```python
from build123d import *

# Parameters (mm, degrees)
SKIZZE1_R                       = 1.75
AUFSATZ_LINEAR_AUSTRAGEN1_DEPTH = 29
SKIZZE2_W                       = 95.177468056
SKIZZE2_H                       = 43
SCHNITT_LINEAR_AUSTRAGEN1_DEPTH = 29
SKIZZE5_W                       = 102.378587485
SKIZZE5_H                       = 44.26226899
SCHNITT_LINEAR_AUSTRAGEN2_DEPTH = 29
SKIZZE6_W                       = 21
SKIZZE6_H                       = 11
SCHNITT_LINEAR_AUSTRAGEN3_DEPTH = 2
SKIZZE7_R                       = 3
SCHNITT_LINEAR_AUSTRAGEN4_DEPTH = 2
SKIZZE8_R                       = 1.75
SCHNITT_LINEAR_AUSTRAGEN5_DEPTH = 102.965680501


with BuildPart() as part:
    # Skizze1 → Aufsatz-Linear austragen1 (new body)
    with BuildSketch(Plane.XY):
        with BuildLine():
            Line((31, -13.5), (31, 0.5))
            ThreePointArc((31, 0.5), (30.121320344, 2.621320344), (28, 3.5))
            Line((28, 3.5), (-15, 3.5))
            ThreePointArc((-15, 3.5), (-21.363961031, 6.136038969), (-24, 12.5))
            Line((-24, 12.5), (-24, 30.5))
            ThreePointArc((-24, 30.5), (-24.878679656, 32.621320344), (-27, 33.5))
            Line((-27, 33.5), (-81, 33.5))
            ThreePointArc((-81, 33.5), (-83.121320344, 32.621320344), (-84, 30.5))
            Line((-84, 30.5), (-84, 29.5))
            ThreePointArc((-84, 29.5), (-83.121320344, 27.378679656), (-81, 26.5))
            Line((-81, 26.5), (-36, 26.5))
            ThreePointArc((-36, 26.5), (-32.464466094, 25.035533906), (-31, 21.5))
            Line((-31, 21.5), (-31, 5.5))
            ThreePointArc((-31, 5.5), (-28.363961031, -0.863961031), (-22, -3.5))
            Line((-22, -3.5), (18, -3.5))
            ThreePointArc((18, -3.5), (20.121320344, -4.378679656), (21, -6.5))
            Line((21, -6.5), (21, -13.5))
            ThreePointArc((21, -13.5), (21.878679656, -15.621320344), (24, -16.5))
            Line((24, -16.5), (28, -16.5))
            ThreePointArc((28, -16.5), (30.121320344, -15.621320344), (31, -13.5))
        make_face()
        with Locations(Location((26, -1.150447614, 0), (0, 0, 180))):
            Circle(SKIZZE1_R, mode=Mode.SUBTRACT)
        with Locations(Location((26, -11.849552386, 0), (0, 0, 180))):
            Circle(SKIZZE1_R, mode=Mode.SUBTRACT)
    extrude(amount=AUFSATZ_LINEAR_AUSTRAGEN1_DEPTH)

    # Skizze2 → Schnitt-Linear austragen1 (cut)
    with BuildSketch(Plane.XY.offset(24.5)):
        with Locations((-3.395581908, 5)):
            Rectangle(SKIZZE2_W, SKIZZE2_H)
    extrude(amount=SCHNITT_LINEAR_AUSTRAGEN1_DEPTH, mode=Mode.SUBTRACT)

    # Skizze5 → Schnitt-Linear austragen2 (cut)
    with BuildSketch(Plane.XY.offset(17.5)):
        with Locations((-5.60029533, 4.368865505)):
            Rectangle(SKIZZE5_W, SKIZZE5_H)
    extrude(amount=-SCHNITT_LINEAR_AUSTRAGEN2_DEPTH, mode=Mode.SUBTRACT)

    # Skizze6 → Schnitt-Linear austragen3 (cut)
    with BuildSketch(Plane(origin=(0, 33.5, 0), x_dir=(1, 0, 0), z_dir=(0, 1, 0))):
        with Locations((-54, -7.342518692)):
            Rectangle(SKIZZE6_W, SKIZZE6_H)
        with Locations((-54, -21.657481308)):
            Rectangle(SKIZZE6_W, SKIZZE6_H)
    extrude(amount=-SCHNITT_LINEAR_AUSTRAGEN3_DEPTH, mode=Mode.SUBTRACT)

    # Skizze7 → Schnitt-Linear austragen4 (cut)
    with BuildSketch(Plane.XY.offset(24.5)):
        with Locations((26, -1.150447614)):
            Circle(SKIZZE7_R)
        with Locations((26, -11.849552386)):
            Circle(SKIZZE7_R)
    extrude(amount=-SCHNITT_LINEAR_AUSTRAGEN4_DEPTH, mode=Mode.SUBTRACT)

    # Skizze8 → Schnitt-Linear austragen5 (cut, through all)
    with BuildSketch(Plane(origin=(0, 33.5, 0), x_dir=(1, 0, 0), z_dir=(0, 1, 0))):
        with Locations(Location((-54, -7.342518692, 0), (0, 0, 270))):
            Circle(SKIZZE8_R)
        with Locations(Location((-54, -21.657481308, 0), (0, 0, 90))):
            Circle(SKIZZE8_R)
    extrude(amount=-SCHNITT_LINEAR_AUSTRAGEN5_DEPTH, mode=Mode.SUBTRACT)


solid = part.part
```
For this review, take the finished solid that the model builds, in its own axes (mm). A direction names the side the tool comes from. Give positions to 0.01 mm unless a question says otherwise; leave off trailing zeros. Order: outer loops, then holes, each group sorted by start corner. A loop starts at its lowest first (then second) coordinate and runs counter-clockwise, first axis right, second up.
1) Take a section at D-D (y = 28). Give the boundary of the cut face in (x, z).
2) For faces 1 (the face through (-54, 33.5, 14)), 2 (the face through (26, -3.1, 22.5)), 3 (the face through (-31, 14, 21)), 4 (the face through (-64.5, 33, 22)), list the 3-axis set-ups (+Z, -Z, +X, -X, +Y, -Y) from which the entire face can be reached by the end or side of a thin tool; tool diameter is ignored.
3) Take a section at B-B (z = 7.25). Give the boundary of the cut face in (x, y).
4) The part is to be moulded in two halves that separate along X. For faces 5 (the face through (-43.5, 33, 7)), 6 (the face through (7, 3.5, 21)), 7 (the face through (-83.1, 32.64, 14.3)), say which applies: released by +X, released by -X, zero draft, split by the parting line, or undercut.
5) Take a section at A-A (x = 26). Give the boundary of the cut face in (y, z).
6) Wall thickness on line 1 (Y direction, x = 26, z = 19.45); line 2 (Y direction, x = 26, z = 23.9); line 3 (Z direction, x = -28, y = 5.5): over which ranges is each line inside the solid? List them lowest first.
7) Take a section at C-C (x = -54). Give the boundary of the cut face in (y, z), then the cut area to 3 significant figures.
8) Insertion check: pin 1 (1.5 mm diameter, centred on x = -67, z = 17.5, fed in from -Y); pin 2 (6 mm diameter, centred on x = -30, y = 8, fed in from -Z); pin 3 (5 mm diameter, centred on y = 24.5, z = 21, fed in from -X). Each pin has a flat end and moves straight along its axis. Give the tip position at first contact, or say it passes through.
Derived:
1. outline: (-83.6, 0) - (-24, 0) - (-24, 29) - (-83.6, 29) - close; hole circle Ø3.5 at (-54, 7.34); hole circle Ø3.5 at (-54, 21.66)
2. face 1: +Z, -Z, +X, -X, +Y
2. face 2: +Z
2. face 3: +Z, -Z, -X, -Y
2. face 4: +Y
3. outline: (-84, 29.5) arc R3 ccw to (-81, 26.5) - (-55.75, 26.5) - (-55.75, 31.5) - (-64.5, 31.5) - (-64.5, 33.5) - (-81, 33.5) arc R3 ccw to (-84, 30.5) - close; (-52.25, 26.5) - (-24, 26.5) - (-24, 30.5) arc R3 ccw to (-27, 33.5) - (-43.5, 33.5) - (-43.5, 31.5) - (-52.25, 31.5) - close
4. face 5: undercut
4. face 6: zero draft
4. face 7: released by -X
5. outline: (-16.5, 17.5) - (-13.6, 17.5) - (-13.6, 22.5) - (-14.85, 22.5) - (-14.85, 24.5) - (-16.5, 24.5) - close; (-10.1, 17.5) - (-2.9, 17.5) - (-2.9, 22.5) - (-4.15, 22.5) - (-4.15, 24.5) - (-8.85, 24.5) - (-8.85, 22.5) - (-10.1, 22.5) - close; (0.6, 17.5) - (3.5, 17.5) - (3.5, 24.5) - (1.85, 24.5) - (1.85, 22.5) - (0.6, 22.5) - close
6. line 1: y = -16.5 to -13.6, -10.1 to -2.9, 0.6 to 3.5
6. line 2: y = -16.5 to -14.85, -8.85 to -4.15, 1.85 to 3.5
6. line 3: z = 17.5 to 24.5
7. outline: (26.5, 0) - (33.5, 0) - (33.5, 1.84) - (31.5, 1.84) - (31.5, 5.59) - (26.5, 5.59) - close; (26.5, 9.09) - (31.5, 9.09) - (31.5, 12.84) - (33.5, 12.84) - (33.5, 16.16) - (31.5, 16.16) - (31.5, 19.91) - (26.5, 19.91) - close; (26.5, 23.41) - (31.5, 23.41) - (31.5, 27.16) - (33.5, 27.16) - (33.5, 29) - (26.5, 29) - close
7. area: 124 mm2
8. pin 1: stops at y = 26.5
8. pin 2: stops at z = 17.5
8. pin 3: stops at x = -82.66
